from build123d import *

# Parameters (mm, degrees)
BOSS_EXTRUDE1_DEPTH                 = 139.7
F_5_32_0_15625_DIAMETER_HOLE1_D     = 3.96875
F_5_32_0_15625_DIAMETER_HOLE1_DEPTH = 38.100461051
FILLET1_R                           = 0.381
FILLET2_R                           = 0.7874


with BuildPart() as part:
    # Sketch1 → Boss-Extrude1 (new body)
    with BuildSketch(Plane.XY):
        with BuildLine():
            Line((62.610769474, -36.322), (50.8, -36.322))
            Line((50.8, -36.322), (50.8, 0))
            Line((50.8, 0), (-50.8, 0))
            Line((-50.8, 0), (-50.8, -36.322))
            Line((-50.8, -36.322), (-62.610769474, -36.322))
            ThreePointArc((-62.610769474, -36.322), (-63.5, -37.211230526), (-62.610769474, -38.100461051))
            Line((-62.610769474, -38.100461051), (-49.276, -38.100461051))
            Line((-49.276, -38.100461051), (-49.276, -5.080461051))
            Line((-49.276, -5.080461051), (-40.7924, -5.080461051))
            Line((-40.7924, -5.080461051), (-40.7924, -36.576461051))
            ThreePointArc((-40.7924, -36.576461051), (-40.0304, -37.338461051), (-39.2684, -36.576461051))
            Line((-39.2684, -36.576461051), (-39.2684, -5.080461051))
            Line((-39.2684, -5.080461051), (-30.7848, -5.080461051))
            Line((-30.7848, -5.080461051), (-30.7848, -36.576461051))
            ThreePointArc((-30.7848, -36.576461051), (-30.0228, -37.338461051), (-29.2608, -36.576461051))
            Line((-29.2608, -36.576461051), (-29.2608, -5.080461051))
            Line((-29.2608, -5.080461051), (-20.7772, -5.080461051))
            Line((-20.7772, -5.080461051), (-20.7772, -36.576461051))
            ThreePointArc((-20.7772, -36.576461051), (-20.0152, -37.338461051), (-19.2532, -36.576461051))
            Line((-19.2532, -36.576461051), (-19.2532, -5.080461051))
            Line((-19.2532, -5.080461051), (-10.7696, -5.080461051))
            Line((-10.7696, -5.080461051), (-10.7696, -36.576461051))
            ThreePointArc((-10.7696, -36.576461051), (-10.0076, -37.338461051), (-9.2456, -36.576461051))
            Line((-9.2456, -36.576461051), (-9.2456, -5.080461051))
            Line((-9.2456, -5.080461051), (-0.762, -5.080461051))
            Line((-0.762, -5.080461051), (-0.762, -36.576461051))
            ThreePointArc((-0.762, -36.576461051), (0, -37.338461051), (0.762, -36.576461051))
            Line((0.762, -36.576461051), (0.762, -5.080461051))
            Line((0.762, -5.080461051), (9.2456, -5.080461051))
            Line((9.2456, -5.080461051), (9.2456, -36.576461051))
            ThreePointArc((9.2456, -36.576461051), (10.0076, -37.338461051), (10.7696, -36.576461051))
            Line((10.7696, -36.576461051), (10.7696, -5.080461051))
            Line((10.7696, -5.080461051), (19.2532, -5.080461051))
            Line((19.2532, -5.080461051), (19.2532, -36.576461051))
            ThreePointArc((19.2532, -36.576461051), (20.0152, -37.338461051), (20.7772, -36.576461051))
            Line((20.7772, -36.576461051), (20.7772, -5.080461051))
            Line((20.7772, -5.080461051), (29.2608, -5.080461051))
            Line((29.2608, -5.080461051), (29.2608, -36.576461051))
            ThreePointArc((29.2608, -36.576461051), (30.0228, -37.338461051), (30.7848, -36.576461051))
            Line((30.7848, -36.576461051), (30.7848, -5.080461051))
            Line((30.7848, -5.080461051), (39.2684, -5.080461051))
            Line((39.2684, -5.080461051), (39.2684, -36.576461051))
            ThreePointArc((39.2684, -36.576461051), (40.0304, -37.338461051), (40.7924, -36.576461051))
            Line((40.7924, -36.576461051), (40.7924, -5.080461051))
            Line((40.7924, -5.080461051), (49.276, -5.080461051))
            Line((49.276, -5.080461051), (49.276, -38.100461051))
            Line((49.276, -38.100461051), (62.610769474, -38.100461051))
            ThreePointArc((62.610769474, -38.100461051), (63.5, -37.211230526), (62.610769474, -36.322))
        make_face()
    extrude(amount=-BOSS_EXTRUDE1_DEPTH)

    # 5/32 (0.15625) Diameter Hole1
    with Locations(Plane(origin=(0, -38.100461051, 0), x_dir=(-1, 0, 0), z_dir=(0, -1, 0))):
        with Locations((56.388, 6.35), (56.388, 69.85), (56.388, 133.35), (-56.388, 6.35), (-56.388, 69.85), (-56.388, 133.35)):
            Hole(F_5_32_0_15625_DIAMETER_HOLE1_D / 2, depth=F_5_32_0_15625_DIAMETER_HOLE1_DEPTH)

    # Fillet1
    fillet1_edges = [part.edges().sort_by_distance(p)[0] for p in [
        (-50.8, 0, -69.85),
        (50.8, 0, -69.85),
    ]]
    fillet(fillet1_edges, radius=FILLET1_R)

    # Fillet2
    fillet2_edges = [part.edges().sort_by_distance(p)[0] for p in [
        (49.276, -38.100461051, -69.85),
        (49.276, -5.080461051, -69.85),
        (40.7924, -5.080461051, -69.85),
        (39.2684, -5.080461051, -69.85),
        (30.7848, -5.080461051, -69.85),
        (29.2608, -5.080461051, -69.85),
        (20.7772, -5.080461051, -69.85),
        (19.2532, -5.080461051, -69.85),
        (10.7696, -5.080461051, -69.85),
        (9.2456, -5.080461051, -69.85),
        (0.762, -5.080461051, -69.85),
        (-0.762, -5.080461051, -69.85),
        (-9.2456, -5.080461051, -69.85),
        (-10.7696, -5.080461051, -69.85),
        (-19.2532, -5.080461051, -69.85),
        (-20.7772, -5.080461051, -69.85),
        (-29.2608, -5.080461051, -69.85),
        (-30.7848, -5.080461051, -69.85),
        (-39.2684, -5.080461051, -69.85),
        (-40.7924, -5.080461051, -69.85),
        (-49.276, -5.080461051, -69.85),
        (-49.276, -38.100461051, -69.85),
        (-50.8, -36.322, -69.85),
        (50.8, -36.322, -69.85),
    ]]
    fillet(fillet2_edges, radius=FILLET2_R)


solid = part.part
For this review, take the finished solid that the model builds, in its own axes (mm). A direction names the side the tool comes from. Give positions to 0.01 mm unless a question says otherwise; leave off trailing zeros. Order: outer loops, then holes, each group sorted by start corner. A loop starts at its lowest first (then second) coordinate and runs counter-clockwise, first axis right, second up. Notation, with made-up numbers: M -31,-32 L 18,-32 A20 cw 18,6 Z; hole C 74.25,85.5 d3. An arc over 180 degrees is marked long. Answer in a Markdown table with one row per item. Add a question column.
(1) Wall thickness on probe 1 along X at (y, z) = (-37.4, -133.35); probe 2 along Y at (x, z) = (33, -113); probe 3 along Y at (x, z) = (-52, -28.5): over which ranges is each line inside the solid? List them lowest first. Write a range as [from, to].
(2) Consider section C-C on y = -3.5. State the section outline as (x, z) points, and give its area (3 significant figures).
(3) Consider section D-D on x = -35.5. State the section outline as (y, z) points, and give its area (3 significant figures).
(4) Consider section A-A on y = -20. Give the number of separate pieces and of enclosed holes in the cut face, and give its area (3 significant figures).
(5) For faces 1 (the face through (57.304, -37.199, -131.59)), 2 (the face through (58.4, -36.322, -68.9)), 3 (the face through (25, -5.08, -69)), list the 3-axis set-ups (+Z, -Z, +X, -X, +Y, -Y) from which the entire face can be reached by the end or side of a thin tool; tool diameter is ignored.
(6) Mouldability with a two-part tool opening along X and no side actions: class faces 4 (the face through (-50.8, -18, -69)), 5 (the face through (-39.268, -21, -69)), 6 (the face through (-59, -38.1, -69)) as +X half, -X half, draft (parallel to the pull), parting line (faces both ways), or undercut.
(7) For pin 1 (10 mm diameter, centred on y = -26, z = -91.5, fed in from +X); pin 2 (8 mm diameter, centred on y = -32.5, z = -30, fed in from +X); pin 3 (9 mm diameter, centred on y = -26, z = -101.5, fed in from -X); pin 4 (8 mm diameter, centred on x = 16.5, y = -32, fed in from -Z), all flat-tipped, find the tip position at first contact; note any pin that passes through.
Evaluation:
| question | item | result |
|---|---|---|
| 1 | probe 1 | x = [-63.48, -58.37], [-54.4, -49.28], [49.28, 54.4], [58.37, 63.48] |
| 1 | probe 2 | y = [-5.08, 0] |
| 1 | probe 3 | y = [-38.1, -36.32] |
| 2 | outline | M -50.8,-139.7 L 50.8,-139.7 L 50.8,0 L -50.8,0 Z |
| 2 | area | 14,200 mm^2 |
| 3 | outline | M -5.08,-139.7 L 0,-139.7 L 0,0 L -5.08,0 Z |
| 3 | area | 710 mm^2 |
| 4 | separate pieces | 11 |
| 4 | enclosed holes | 0 |
| 4 | area | 2,340 mm^2 |
| 5 | face 1 | +Y, -Y |
| 5 | face 2 | +Z, -Z, +X, +Y |
| 5 | face 3 | +Z, -Z, -Y |
| 6 | face 4 | -X half |
| 6 | face 5 | undercut |
| 6 | face 6 | draft |
| 7 | pin 1 | stops at x = 50.8 |
| 7 | pin 2 | stops at x = 63.14 |
| 7 | pin 3 | stops at x = -50.8 |
| 7 | pin 4 | stops at z = -139.7 |
